CAD build for the part. Positions are in the model's coordinates, mm. A direction names the side the tool comes from. Give positions to 0.01 mm unless a question says otherwise; leave off trailing zeros. Write each loop counter-clockwise with the first axis right and the second up, starting at its lowest first coordinate (ties: lowest second). Pieces come first, ordered by that corner, then holes. Notation, with made-up numbers: (-16.5, -11.5) - (1.5, -11.5) arc R26 cw to (1.5, 2.5) - close; hole circle Ø4 at (-11, -25). An arc over 180 degrees is marked (long way). Put each result on its own line as item: value. Start each with the question number.
1. Drop flat-ended pins along their axis: pin 1 (1.5 mm diameter, centred on x = 1, y = -14, fed in from -Z); pin 2 (1 mm diameter, centred on y = 2, z = -1, fed in from +X). Give the stop position or say it passes through.
2. Mould opens along Y. For faces 3 (the flat face through (0, -21, 0)), 4 (the cylindrical face through (0.7, -18.82, 0.91)), 5 (the cylindrical face through (1.5, 11.85, -0.07)) say: +Y half, -Y half, draft (parallel to the pull), parting line (faces both ways), or undercut.
3. Cut at A-A on y = 0. List the corners of the cut face in (x, z).
4. Wall check: line 1 (Y direction, x = 0.35, z = 1.15); line 2 (X direction, y = -8, z = 0.75); line 3 (X direction, y = -13.5, z = 0.6). Give the ranges that are in metal, low to high.
5. Tool access for faces 1 (the cylindrical face through (1.5, -8.15, -0.07)), 2 (the cylindrical face through (0.7, 2.83, 0.91)): list every direction of +Z, -Z, +X, -X, +Y, -Y with a clear straight run to the whole face (end or side of a thin tool).
Autodesk Inventor part; units mm, degrees
ref_plane "YZ Plane" through (0, 0, 0) normal (1, 0, 0) x (0, 1, 0)
ref_plane "XZ Plane" through (0, 0, 0) normal (0, 1, 0) x (-1, 0, 0)
ref_plane "XY Plane" through (0, 0, 0) normal (0, 0, 1) x (1, 0, 0)
sketch "Sketch4" plane through (0, 0, 0) normal (0, 1, 0) x (-1, 0, 0)
  circle A0 centre (0, 0) radius 1.5
extrude "Extrusion2" add sketch "Sketch4" along normal mid plane 42
thread "Thread1"
chamfer "Chamfer1" distance 0.2 angle 45 2 edges at (1.5, 21, 0) (1.5, -21, 0)
sketch "Sketch14" plane through (0, 0, 0) normal (1, 0, 0) x (0, 1, 0)
  line L0 (-20.8, -1.5) -> (20.8, -1.5)
  line L1 (3.15, -1.5) -> (2.5, -1.5)
  line L2 (2.5, -1.5) -> (2.5, -1.15)
  line L3 (2.5, -1.15) -> (3.15, -1.15)
  line L4 (3.15, -1.15) -> (3.15, -1.5)
  line L5 (-21, -1.3) -> (-21, 1.3)
  line L6 (-21, 0) -> (13, 0) construction
  line L7 (-20.8, -1.5) -> (20.8, -1.5)
  line L8 (-18.5, -1.5) -> (-19.15, -1.5)
  line L9 (-19.15, -1.5) -> (-19.15, -1.15)
  line L10 (-19.15, -1.15) -> (-18.5, -1.15)
  line L11 (-18.5, -1.15) -> (-18.5, -1.5)
  point P0 (0, 0)
  point P1 (-19.15, -1.5)
  dimension "d105" = 1.15
  dimension "d106" = 0.65
  dimension "d107" = 23.5
  dimension "d109" = 0.65
  dimension "d110" = 1.15
  dimension "d111" = 21
revolve "Revolution1" cut sketch "Sketch14" angle 360 about axis through (0, -21, 0) along (0, 1, 0)
equation "\"d109\" = d106"
equation "\"d110\" = d105"
properties part number "Ball Track Support" material "Bronze, Soft Tin"
Report:
1. pin 1: stops at z = -1.48
1. pin 2: stops at x = 1.41
2. face 3: -Y half
2. face 4: undercut
2. face 5: draft
3. outline: circle Ø3 at (0, 0)
4. line 1: y = -21 to -19.15, -18.5 to 2.5, 3.15 to 21
4. line 2: x = -1.3 to 1.3
4. line 3: x = -1.37 to 1.37
5. face 1: +Y, -Y
5. face 2: none
